Answer from the drawing. Dimensions are ordinates in mm from the lowest x, y and z of the part. A direction names the side the tool comes from. Coordinates: 2 decimals unless noted, no trailing zeros. Order: outer loops, then holes, each group sorted by start corner. A loop starts at its lowest first (then second) coordinate and runs counter-clockwise, first axis right, second up. Notation, with made-up numbers: (85.25, -39.75) -> (90.25, -39.75) arc R28 cw to (90.25, -6.75) -> close; hole circle Ø5 at (-22.75, -22.75). An arc over 180 degrees is marked (long way). Answer in a Markdown table with one row per item.
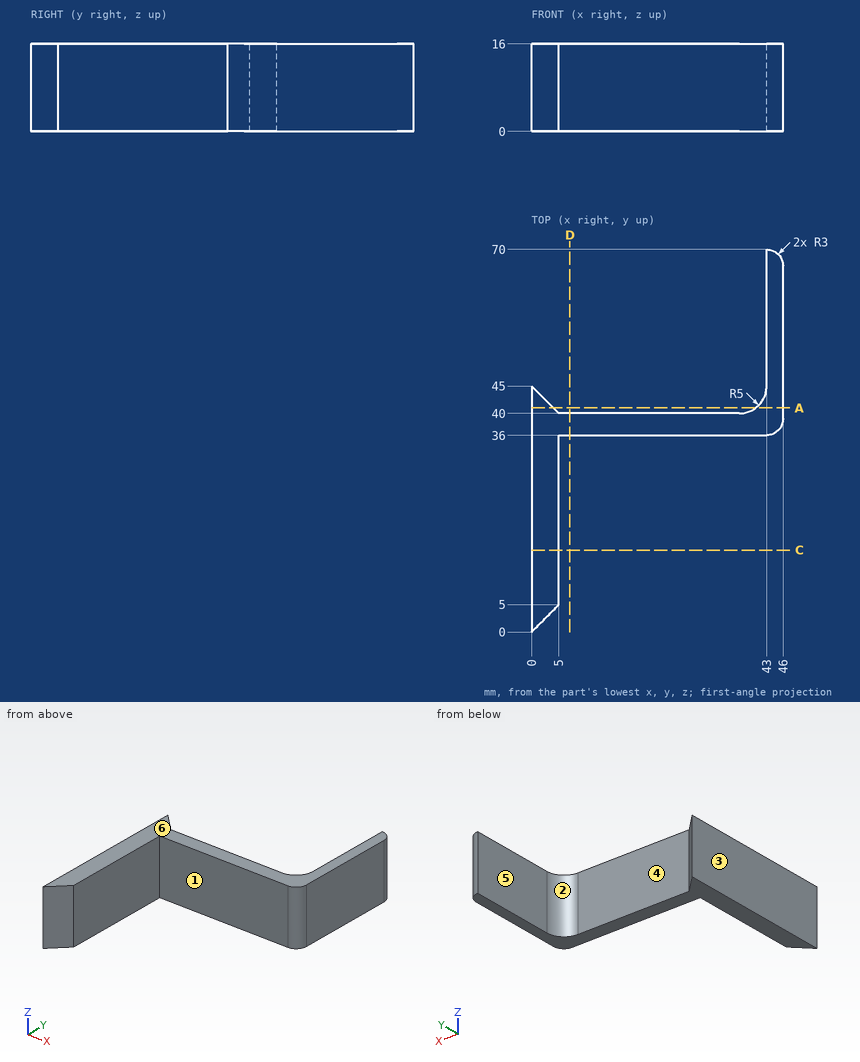
Q1. For the marked faces 1, 2 and 3, determine the directions among +Z, -Z, +X, -X, +Y, -Y from which every point of the face is accessible in a straight line to the end or side of a thin tool.
Outcome:
| item | result |
|---|---|
| face 1 | +Z, -Z, +X, -Y |
| face 2 | +Z, -Z, +Y |
| face 3 | +Z, -Z, -X, +Y, -Y |
Q2. The part is cut by section A-A (y = 41). Write down the section's boundary in (x, z), then the cut area to 3 significant figures.
Outcome:
| item | result |
|---|---|
| outline | (0, 0) -> (4, 0) -> (4, 16) -> (0, 16) -> close; (41, 0) -> (46, 0) -> (46, 16) -> (41, 16) -> close |
| area | 144 mm² |
Q3. Consider line 1 (X direction, y = 23, z = 13.75); line 2 (X direction, y = 60.5, z = 2.5); line 3 (Y direction, x = 10.5, z = 13.5). Determine where each line is inside the solid, lowest interval first.
Outcome:
| item | result |
|---|---|
| line 1 | 0 to 5 |
| line 2 | 43 to 46 |
| line 3 | 36 to 40 |
Q4. The part is cut by section D-D (x = 7). Write down the section's boundary in (y, z).
Outcome:
| item | result |
|---|---|
| outline | (36, 0) -> (40, 0) -> (40, 16) -> (36, 16) -> close |
Q5. Given pin 1 (5 mm diameter, centred on x = 5, z = 6, fed in from -Y); pin 2 (2 mm diameter, centred on x = 33.5, z = 5, fed in from -Y); pin 3 (1.5 mm diameter, centred on x = 15.5, z = 9, fed in from +Y), each flat-ended and moving along its own axis, determine where each tip first touches the part or whether it passes through.
Outcome:
| item | result |
|---|---|
| pin 1 | y = 2.5 |
| pin 2 | y = 36 |
| pin 3 | y = 40 |
Q6. The part is cut by section C-C (y = 15). Write down the section's boundary in (x, z), then the cut area to 3 significant figures.
Outcome:
| item | result |
|---|---|
| outline | (0, 0) -> (5, 0) -> (5, 16) -> (0, 16) -> close |
| area | 80.0 mm² |
Q7. For a pull along X with two mould halves and no side action, classify the marked faces 4, 5 and 6 as pulls with the +X half, pulls with the -X half, needs draft (parallel to the pull), parting line crosses it, or undercut.
Outcome:
| item | result |
|---|---|
| face 4 | undercut |
| face 5 | pulls with the -X half |
| face 6 | needs draft |
